The model under review builds one solid part; all positions refer to its coordinate system, in mm. A direction names the side the tool comes from. Round coordinates to 2 decimals unless told otherwise and drop trailing zeros. Loops run counter-clockwise (first coordinate to the right, second up) from the corner with the lowest first, then second, coordinate; pieces in that order, holes last. Notation, with made-up numbers: (67, -3.75) -> (113, -3.75) arc R29 ccw to (113, 16.25) -> close; hole circle Ø9 at (-31.75, -8.5). An arc over 180 degrees is marked (long way). Use a Markdown table: item, result. Add a question column.
1) Consider section D-D on z = -3.75. Give the boundary of the cut face in (x, y), plus the area to 3 significant figures.
2) Consider section B-B on y = 20. Give the boundary of the cut face in (x, z), plus the area to 3 significant figures.
3) Mouldability with a two-part tool opening along X and no side actions: class faces 4 (the flat face through (101, 3, -3)), 5 (the flat face through (0, 34, -10)), 6 (the flat face through (154.955, 56.065, -9.86)) as released by +X, released by -X, zero draft, split by the parting line, or undercut.
4) Consider section A-A on z = -16.75. Give the boundary of the cut face in (x, y), plus the area to 3 significant figures.
5) Consider section C-C on x = 16. Give the boundary of the cut face in (y, z), plus the area to 3 significant figures.
6) For faces 1 (the flat face through (137, 15, -10)), 2 (the flat face through (28, 3, -3)), 3 (the flat face through (65, 6, -17)), list the 3-axis set-ups (+Z, -Z, +X, -X, +Y, -Y) from which the entire face can be reached by the end or side of a thin tool; tool diameter is ignored.
7) Insertion check: pin 1 (10 mm diameter, centred on x = 150, z = -5, fed in from +Y); pin 2 (5 mm diameter, centred on x = 58, z = -17.5, fed in from -Y); pin 3 (3 mm diameter, centred on x = 55.5, y = 3.5, fed in from -Z); pin 4 (9.5 mm diameter, centred on x = 15, y = 20, fed in from -Z). Each pin has a flat end and moves straight along its axis. Give the tip position at first contact, or say it passes through.
8) Wall thickness on probe 1 along X at (y, z) = (25.5, -17); probe 2 along Y at (x, z) = (114, -5.5); probe 3 along Y at (x, z) = (15, -4.5): over which ranges is each line inside the solid? List them lowest first.
Solid Edge part; units mm, degrees
sketch "Sketch1" plane through (0, 0, 0) normal (0, 0, 1) x (1, 0, 0)
  line L0 (0, 0) -> (173.42, 0)
  line L1 (173.42, 0) -> (173.42, 82.87)
  line L2 (173.42, 82.87) -> (0, 82.87)
  line L3 (0, 82.87) -> (0, 0)
extrude "Protrusion1" add sketch "Sketch1" against normal blind 20
sketch "Sketch2" plane through (86.71, 41.435, 0) normal (0, 0, 1) x (0, 1, 0)
  line L0 (-41.435, -50.29) -> (-11.435, -50.29)
  line L1 (-11.435, -50.29) -> (41.435, -86.71)
  line L2 (41.435, -86.71) -> (-41.435, -86.71)
  line L3 (-41.435, -86.71) -> (-41.435, -50.29)
extrude "ExtrudedCutout_1" cut sketch "Sketch2" against normal blind 20
sketch "Sketch3" plane through (86.71, 41.435, 0) normal (0, 0, 1) x (0, 1, 0)
  line L0 (25.565, 86.71) -> (41.435, -86.71)
  line L1 (41.435, -86.71) -> (41.435, 86.71)
  line L2 (41.435, 86.71) -> (25.565, 86.71)
extrude "ExtrudedCutout_2" cut sketch "Sketch3" against normal blind 20
sketch "Sketch4" plane through (86.71, 41.435, 0) normal (0, 0, 1) x (1, 0, 0)
  circle A0 centre (-71.71, -21.435) radius 8
  circle A1 centre (27.29, -21.435) radius 8
extrude "ExtrudedCutout_3" cut sketch "Sketch4" against normal blind 20
sketch "Sketch5" plane through (68.5, 0, -10) normal (0, -1, 0) x (1, 0, 0)
  line L0 (35.5, 10) -> (-43.5, 10)
  line L1 (-43.5, 10) -> (-37.5, 4)
  line L2 (29.5, 4) -> (-37.5, 4)
  line L3 (35.5, 10) -> (29.5, 4)
extrude "ExtrudedCutout_4" cut sketch "Sketch5" against normal blind 6
sketch "Sketch6" plane through (68.5, 0, -10) normal (0, -1, 0) x (1, 0, 0)
  line L0 (35.5, -10) -> (-43.5, -10)
  line L1 (35.5, -10) -> (29.5, -4)
  line L2 (29.5, -4) -> (-37.5, -4)
  line L3 (-43.5, -10) -> (-37.5, -4)
extrude "ExtrudedCutout_5" cut sketch "Sketch6" against normal blind 6
Result set:
| question | item | result |
|---|---|---|
| 1 | outline | (0, 0) -> (28.75, 0) -> (28.75, 6) -> (100.25, 6) -> (100.25, 0) -> (137, 0) -> (137, 30) -> (173.42, 82.87) -> (0, 67) -> close; hole circle Ø16 at (15, 20); hole circle Ø16 at (114, 20) |
| 1 | area | 10,100 mm2 |
| 2 | outline | (0, -20) -> (7, -20) -> (7, 0) -> (0, 0) -> close; (23, -20) -> (106, -20) -> (106, 0) -> (23, 0) -> close; (122, -20) -> (137, -20) -> (137, 0) -> (122, 0) -> close |
| 2 | area | 2,100 mm2 |
| 3 | face 4 | undercut |
| 3 | face 5 | released by -X |
| 3 | face 6 | released by +X |
| 4 | outline | (0, 0) -> (28.25, 0) -> (28.25, 6) -> (100.75, 6) -> (100.75, 0) -> (137, 0) -> (137, 30) -> (173.42, 82.87) -> (0, 67) -> close; hole circle Ø16 at (15, 20); hole circle Ø16 at (114, 20) |
| 4 | area | 10,100 mm2 |
| 5 | outline | (0, -20) -> (12.06, -20) -> (12.06, 0) -> (0, 0) -> close; (27.94, -20) -> (68.46, -20) -> (68.46, 0) -> (27.94, 0) -> close |
| 5 | area | 1,050 mm2 |
| 6 | face 1 | +Z, -Z, +X, -Y |
| 6 | face 2 | +Z, -Y |
| 6 | face 3 | -Z, -Y |
| 7 | pin 1 | y = 81.18 |
| 7 | pin 2 | y = 6 |
| 7 | pin 3 | z = -14 |
| 7 | pin 4 | through |
| 8 | probe 1 | 0 to 9.19, 20.81 to 108.19, 119.81 to 137 |
| 8 | probe 2 | 0 to 12, 28 to 77.43 |
| 8 | probe 3 | 0 to 12, 28 to 68.37 |
